from build123d import *

# Parameters (mm, degrees)
F1_DEPTH = 6.35
F0_R     = 3.175
F2_DEPTH = 2.794
F4_DEPTH = 1.5875
F6_DEPTH = 6.35


with BuildPart() as f1:
    # F0 (on Top) → F1 (new body)
    with BuildSketch(Plane.XY):
        with BuildLine():
            ThreePointArc((13.890625, 23.415625), (0, 37.30625), (-13.890625, 23.415625))
            Line((-13.890625, 23.415625), (-13.890625, -23.415625))
            ThreePointArc((-13.890625, -23.415625), (0, -37.30625), (13.890625, -23.415625))
            Line((13.890625, -23.415625), (13.890625, 23.415625))
        make_face()
    extrude(amount=F1_DEPTH)

    # F0 (on Top) → F2 (join)
    with BuildSketch(Plane.XY):
        with BuildLine():
            ThreePointArc((17.065625, 37.30625), (0, 54.371875), (-17.065625, 37.30625))
            Line((-17.065625, 37.30625), (-17.065625, -37.30625))
            ThreePointArc((-17.065625, -37.30625), (0, -54.371875), (17.065625, -37.30625))
            Line((17.065625, -37.30625), (17.065625, 37.30625))
        make_face()
        with Locations((0, -44.846875)):
            Circle(F0_R, mode=Mode.SUBTRACT)
        with BuildLine():
            Line((-13.890625, -23.415625), (-13.890625, 23.415625))
            ThreePointArc((-13.890625, 23.415625), (0, 37.30625), (13.890625, 23.415625))
            Line((13.890625, 23.415625), (13.890625, -23.415625))
            ThreePointArc((13.890625, -23.415625), (0, -37.30625), (-13.890625, -23.415625))
        make_face(mode=Mode.SUBTRACT)
        with Locations((0, 44.846875)):
            Circle(F0_R, mode=Mode.SUBTRACT)
        with BuildLine():
            ThreePointArc((13.890625, 23.415625), (0, 37.30625), (-13.890625, 23.415625))
            Line((-13.890625, 23.415625), (-13.890625, -23.415625))
            ThreePointArc((-13.890625, -23.415625), (0, -37.30625), (13.890625, -23.415625))
            Line((13.890625, -23.415625), (13.890625, 23.415625))
        make_face()
    extrude(amount=-F2_DEPTH)

    # F3 (on face) → F4 (join)
    with BuildSketch(Plane(origin=(0, 0, -2.794), x_dir=(1, 0, 0), z_dir=(0, 0, -1))):
        with BuildLine():
            ThreePointArc((17.065625, 37.30625), (0, 54.371875), (-17.065625, 37.30625))
            Line((-17.065625, 37.30625), (-17.065625, -37.30625))
            ThreePointArc((-17.065625, -37.30625), (0, -54.371875), (17.065625, -37.30625))
            Line((17.065625, -37.30625), (17.065625, 37.30625))
        make_face()
    extrude(amount=F4_DEPTH)

    # F5 (on face) → F6 (cut, through all)
    with BuildSketch(Plane.XY.offset(6.35)):
        with BuildLine():
            ThreePointArc((10.715625, 23.415625), (0, 34.13125), (-10.715625, 23.415625))
            Line((-10.715625, 23.415625), (-10.715625, -23.415625))
            ThreePointArc((-10.715625, -23.415625), (0, -34.13125), (10.715625, -23.415625))
            Line((10.715625, -23.415625), (10.715625, 23.415625))
        make_face()
    extrude(amount=-F6_DEPTH, mode=Mode.SUBTRACT)


solid = f1.part
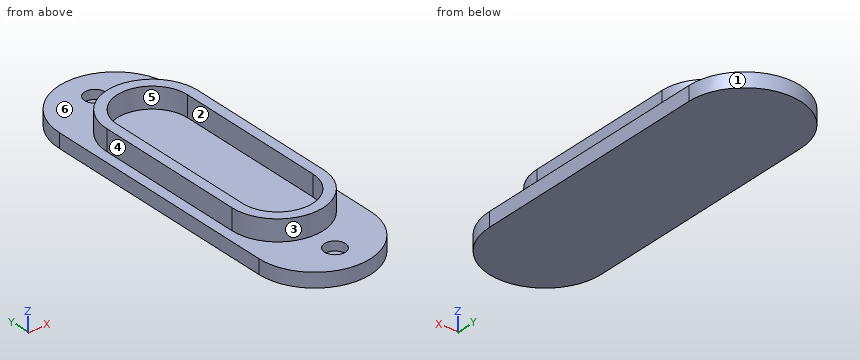
Build history of the part. All positions in model axes, mm. Face numbers are marked on the shaded views. A direction names the side the tool comes from. Coordinates: 2 decimals unless noted, no trailing zeros. Order: outer loops, then holes, each group sorted by start corner. A loop starts at its lowest first (then second) coordinate and runs counter-clockwise, first axis right, second up. Notation, with made-up numbers: (-34.5, 0.5) - (-21.5, 0.5) arc R27 cw to (-21.5, 30.5) - close; hole circle Ø3 at (22, -2). An arc over 180 degrees is marked (long way). Write each question's results on one line, items separated by ' | '. Start each with the question number.
Item 1: Flat gauge pins, fed straight in: pin 1 (3 mm diameter, centred on y = 3, z = 4, fed in from +X); pin 2 (3 mm diameter, centred on x = 2, y = 16.5, fed in from +Z); pin 3 (5 mm diameter, centred on y = -7.5, z = 3.5, fed in from -X). Where does each tip first touch, or does it go through?
Item 2: Band-saw the part on C-C on x = 0. Write the cut outline in (y, z), and give its area (3 significant figures).
Item 3: Band-saw the part on B-B on z = 5.25. Write the cut outline in (x, y).
Item 4: Band-saw the part on D-D on y = -26.5. Write the cut outline in (x, z), and give its area (3 significant figures).
Item 5: Mould opens along X. For the marked faces 3, 4, 5 and 6 say: released by +X, released by -X, zero draft, split by the parting line, or undercut.
Item 6: Wall check: probe 1 along Y at (x, z) = (0, -0.8); probe 2 along X at (y, z) = (-6.5, 0.5); probe 3 along Z at (x, y) = (-15.5, -25). Give the ranges that are in metal, low to high. Write a range as [from, to].
Item 7: Tool access for the marked faces 1 and 2: list every direction of +Z, -Z, +X, -X, +Y, -Y with a clear straight run to the whole face (end or side of a thin tool).
Item 8: Band-saw the part on A-A on y = 21. Write the cut outline in (x, z).
Numbers:
1) pin 1: x = 13.89 | pin 2: z = 0 | pin 3: x = -13.89
2) outline: (-54.37, -4.38) - (54.37, -4.38) - (54.37, 0) - (48.02, 0) - (48.02, -2.79) - (41.67, -2.79) - (41.67, 0) - (37.31, 0) - (37.31, 6.35) - (34.13, 6.35) - (34.13, 0) - (-34.13, 0) - (-34.13, 6.35) - (-37.31, 6.35) - (-37.31, 0) - (-41.67, 0) - (-41.67, -2.79) - (-48.02, -2.79) - (-48.02, 0) - (-54.37, 0) - close | area: 481 mm^2
3) outline: (-13.89, -23.42) arc R13.89 ccw to (13.89, -23.42) - (13.89, 23.42) arc R13.89 ccw to (-13.89, 23.42) - close; hole (-10.72, -23.42) arc R10.72 ccw to (10.72, -23.42) - (10.72, 23.42) arc R10.72 ccw to (-10.72, 23.42) - close
4) outline: (-17.07, -4.38) - (17.07, -4.38) - (17.07, 0) - (13.54, 0) - (13.54, 6.35) - (10.26, 6.35) - (10.26, 0) - (-10.26, 0) - (-10.26, 6.35) - (-13.54, 6.35) - (-13.54, 0) - (-17.07, 0) - close | area: 191 mm^2
5) face 3: split by the parting line | face 4: released by -X | face 5: undercut | face 6: zero draft
6) probe 1: [-54.37, -48.02], [-41.67, 41.67], [48.02, 54.37] | probe 2: [-13.89, -10.72], [10.72, 13.89] | probe 3: [-4.38, 0]
7) face 1: +Z, -Z, +Y | face 2: +Z
8) outline: (-17.07, -4.38) - (17.07, -4.38) - (17.07, 0) - (13.89, 0) - (13.89, 6.35) - (10.72, 6.35) - (10.72, 0) - (-10.72, 0) - (-10.72, 6.35) - (-13.89, 6.35) - (-13.89, 0) - (-17.07, 0) - close
